The listing builds one solid part. Answer for the finished solid, in the listing's coordinates (mm). Face numbers are marked on the shaded views. Give positions to 0.01 mm unless a question says otherwise; leave off trailing zeros. Order: outer loops, then holes, each group sorted by start corner. A loop starts at its lowest first (then second) coordinate and runs counter-clockwise, first axis right, second up.
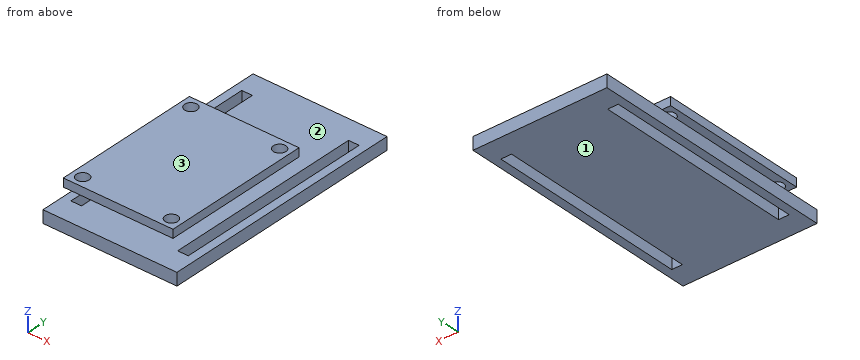
Autodesk Fusion 360 part; units mm, degrees
sketch "Boceto1" plane through (0, 0, 0) normal (0, 0, 1) x (1, 0, 0)
  line L0 (0, 0) -> (30, 0)
  line L1 (30, 0) -> (30, 57)
  line L2 (30, 57) -> (0, 57)
  line L3 (0, 57) -> (0, 0)
  dimension "d1" = 57
  dimension "d2" = 30
extrude "Extruir1" add sketch "Boceto1" along normal blind 3
sketch "Boceto2" plane through (0, 0, 3) normal (0, 0, 1) x (-1, 0, 0)
  line L0 (0, -57) -> (0, 0)
  line L1 (0, 0) -> (-30, 0)
  line L2 (-30, 0) -> (-30, -57)
  line L3 (-30, -57) -> (0, -57)
  line L4 (-0.98, -52.5) -> (-3.52, -52.5)
  line L5 (-3.52, -52.5) -> (-3.52, -4.5)
  line L6 (-3.52, -4.5) -> (-0.98, -4.5)
  line L7 (-0.98, -4.5) -> (-0.98, -52.5)
  line L8 (-15, -57) -> (-15, 0) construction
  line L9 (-26.48, -52.5) -> (-26.48, -4.5)
  line L10 (-29.02, -4.5) -> (-29.02, -52.5)
  line L11 (-29.02, -52.5) -> (-26.48, -52.5)
  line L12 (-26.48, -4.5) -> (-29.02, -4.5)
  point P0 (-0.98, -28.5)
  point P1 (0, -28.5)
  point P2 (-2.25, -52.5)
  point P3 (-27.75, -52.5)
  dimension "d5" = 2.54
  dimension "d6" = 48
  dimension "d7" = 25.5
extrude "Extruir2" cut sketch "Boceto2" against normal through all contours L4 L5 L6 L7 | L9 L10 L11 L12
sketch "Boceto3" plane through (0, 0, 3) normal (0, 0, 1) x (-1, 0, 0)
  line L0 (-0.98, -4.5) -> (-0.98, -52.5)
  line L1 (-0.98, -52.5) -> (-3.52, -52.5)
  line L2 (-3.52, -52.5) -> (-3.52, -4.5)
  line L3 (-3.52, -4.5) -> (-0.98, -4.5)
  line L4 (-26.48, -4.5) -> (-26.48, -52.5)
  line L5 (-26.48, -52.5) -> (-29.02, -52.5)
  line L6 (-29.02, -52.5) -> (-29.02, -4.5)
  line L7 (-29.02, -4.5) -> (-26.48, -4.5)
  line L8 (0, -57) -> (0, 0)
  line L9 (0, 0) -> (-30, 0)
  line L10 (-30, 0) -> (-30, -57)
  line L11 (-30, -57) -> (0, -57)
  line L12 (1, -58) -> (1, 1)
  line L13 (1, 1) -> (-31, 1)
  line L14 (-31, 1) -> (-31, -58)
  line L15 (-31, -58) -> (1, -58)
  dimension "d9" = 1
extrude "Extruir3" add sketch "Boceto3" against normal up to surface (3 mm away) contours L12 L13 L14 L15
sketch "Boceto4" plane through (0, 0, 3) normal (0, 0, 1) x (-1, 0, 0)
  line L0 (-31, -58) -> (1, -58)
  line L1 (1, -58) -> (1, 1)
  line L2 (1, 1) -> (-31, 1)
  line L3 (-31, 1) -> (-31, -58)
  line L4 (-0.98, -4.5) -> (-0.98, -52.5)
  line L5 (-0.98, -52.5) -> (-3.52, -52.5)
  line L6 (-3.52, -52.5) -> (-3.52, -4.5)
  line L7 (-3.52, -4.5) -> (-0.98, -4.5)
  line L8 (-26.48, -4.5) -> (-26.48, -52.5)
  line L9 (-26.48, -52.5) -> (-29.02, -52.5)
  line L10 (-29.02, -52.5) -> (-29.02, -4.5)
  line L11 (-29.02, -4.5) -> (-26.48, -4.5)
  line L12 (-22, -9) -> (-8, -9)
  line L13 (-8, -9) -> (-8, -29)
  line L14 (-8, -29) -> (-22, -29)
  line L15 (-22, -29) -> (-22, -9)
  point P0 (-15, -9)
  point P1 (-15, 1)
  dimension "d12" = 10
  dimension "d13" = 20
  dimension "d14" = 14
extrude "Extruir4" add sketch "Boceto4" along normal blind 5 contours L12 L13 L14 L15
sketch "Boceto5" plane through (0, 0, 8) normal (0, 0, 1) x (-1, 0, 0)
  line L0 (-22, -29) -> (-8, -29)
  line L1 (-8, -29) -> (-8, -9)
  line L2 (-8, -9) -> (-22, -9)
  line L3 (-22, -9) -> (-22, -29)
  line L4 (-28.1, -1.3) -> (-1.9, -1.3)
  line L5 (-1.9, -1.3) -> (-1.9, -36.7)
  line L6 (-1.9, -36.7) -> (-28.1, -36.7)
  line L7 (-28.1, -36.7) -> (-28.1, -1.3)
  line L8 (-25.6, -3.8) -> (-4.4, -3.8)
  line L9 (-4.4, -3.8) -> (-4.4, -34.2)
  line L10 (-4.4, -34.2) -> (-25.6, -34.2)
  line L11 (-25.6, -34.2) -> (-25.6, -3.8)
  circle A0 centre (-25.6, -3.8) radius 1.5
  circle A1 centre (-4.4, -3.8) radius 1.5
  circle A2 centre (-25.6, -34.2) radius 1.5
  circle A3 centre (-4.4, -34.2) radius 1.5
  point P0 (-15, -1.3)
  point P1 (-15, -9)
  point P2 (-1.9, -19)
  point P3 (-8, -19)
  point P4 (-15, -3.8)
  point P5 (-4.4, -19)
  dimension "d17" = 26.2
  dimension "d18" = 35.4
  dimension "d21" = 3
  dimension "d22" = 21.2
  dimension "d23" = 30.4
extrude "Extruir5" add sketch "Boceto5" along normal blind 2 contours L0 L1 L2 L3 | L4 L5 L6 L7 | L8 L9 L10 L11 A0 A1 A2 A3
1) Find section D-D (y = 34.2). Write down the section's boundary in (x, z), then the cut area to 3 significant figures.
Geometry says:
outline: (-1, 0) - (0.98, 0) - (0.98, 3) - (-1, 3) - close; (1.9, 8) - (2.9, 8) - (2.9, 10) - (1.9, 10) - close; (3.52, 0) - (26.48, 0) - (26.48, 3) - (3.52, 3) - close; (5.9, 8) - (24.1, 8) - (24.1, 10) - (5.9, 10) - close; (27.1, 8) - (28.1, 8) - (28.1, 10) - (27.1, 10) - close; (29.02, 0) - (31, 0) - (31, 3) - (29.02, 3) - close
area: 121 mm2
2) Straight lines are drawn through the part: probe 1 along X at (y, z) = (25.5, 1.5); probe 2 along Y at (x, z) = (25.6, 9.2); probe 3 along X at (y, z) = (3.8, 9.05). For each, find the intervals that lie inside material, in ascending order.
Geometry says:
probe 1: x = -1 to 0.98, 3.52 to 26.48, 29.02 to 31
probe 2: y = 1.3 to 2.3, 5.3 to 32.7, 35.7 to 36.7
probe 3: x = 1.9 to 2.9, 5.9 to 24.1, 27.1 to 28.1
3) Find section B-B (z = 9). Write down the section's boundary in (x, y), then the cut area to 3 significant figures.
Geometry says:
outline: (1.9, 1.3) - (28.1, 1.3) - (28.1, 36.7) - (1.9, 36.7) - close; hole circle Ø3 at (4.4, 3.8); hole circle Ø3 at (4.4, 34.2); hole circle Ø3 at (25.6, 3.8); hole circle Ø3 at (25.6, 34.2)
area: 899 mm2
4) Find section A-A (y = 3.8). Write down the section's boundary in (x, z), then the cut area to 3 significant figures.
Geometry says:
outline: (-1, 0) - (31, 0) - (31, 3) - (-1, 3) - close; (1.9, 8) - (2.9, 8) - (2.9, 10) - (1.9, 10) - close; (5.9, 8) - (24.1, 8) - (24.1, 10) - (5.9, 10) - close; (27.1, 8) - (28.1, 8) - (28.1, 10) - (27.1, 10) - close
area: 136 mm2
5) For a pull along Z with two mould halves and no side action, classify the marked faces 1, 2 and 3 as +Z half, -Z half, draft (parallel to the pull), parting line (faces both ways), or undercut.
Geometry says:
face 1: -Z half
face 2: undercut
face 3: +Z half
6) Given P1, Ø1, axis at y = 42.5, z = 4.5, coming from the -X side; P2, Ø5, axis at y = 19, z = 9, coming from the +X side; P3, Ø2.5, axis at x = 4.4, y = 34.2, coming from the +Z side; P4, Ø5, axis at x = 4.5, z = 7.5, coming from the +Y side, each flat-ended and moving along its own axis, determine where each tip first touches the part or whether it passes through.
Geometry says:
P1: passes through
P2: stops at x = 28.1
P3: stops at z = 3
P4: stops at y = 36.7
7) Find section C-C (x = 25.6). Write down the section's boundary in (y, z).
Geometry says:
outline: (-1, 0) - (58, 0) - (58, 3) - (-1, 3) - close; (1.3, 8) - (2.3, 8) - (2.3, 10) - (1.3, 10) - close; (5.3, 8) - (32.7, 8) - (32.7, 10) - (5.3, 10) - close; (35.7, 8) - (36.7, 8) - (36.7, 10) - (35.7, 10) - close
